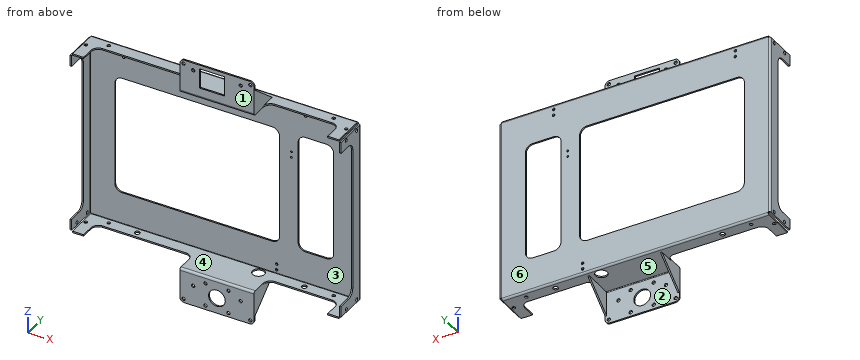
from build123d import *

# Parameters (mm, degrees)
BOSS_EXTRUDE1_DEPTH = 182.5
CUT_EXTRUDE1_DEPTH  = 251
BOSS_EXTRUDE2_START = 17.5
BOSS_EXTRUDE2_DEPTH = 50
BOSS_EXTRUDE3_DEPTH = 2
SKETCH5_R           = 11.25
SKETCH5_R_2         = 2.25
SKETCH5_W           = 34
SKETCH5_H           = 27
CUT_EXTRUDE2_DEPTH  = 2
FILLET1_R           = 10
SKETCH7_W           = 2
SKETCH7_H           = 246
BOSS_EXTRUDE4_DEPTH = 43
SKETCH8_W           = 3
SKETCH8_H           = 3
CUT_EXTRUDE4_DEPTH  = 46
FILLET2_R           = 0.5
FILLET3_R           = 2.5
CUT_EXTRUDE5_DEPTH  = 366
SKETCH10_R          = 2.25
CUT_EXTRUDE6_DEPTH  = 295.5
SKETCH11_R          = 2.25
CUT_EXTRUDE7_DEPTH  = 366
CUT_EXTRUDE8_DEPTH  = 3
SKETCH14_R          = 3.5
SKETCH14_R_2        = 8
CUT_EXTRUDE9_DEPTH  = 10
FILLET4_R           = 6
SKETCH15_R          = 1.75
SKETCH15_R_2        = 1.25
CUT_EXTRUDE10_DEPTH = 10


with BuildPart() as part:
    # Sketch1 → Boss-Extrude1 (new body, symmetric)
    with BuildSketch(Plane(origin=(0, 0, 0), x_dir=(0, 0, -1), z_dir=(1, 0, 0))):
        with BuildLine():
            Line((123, -45), (125, -45))
            Line((125, -45), (125, -2.5))
            ThreePointArc((125, -2.5), (124.267766953, -0.732233047), (122.5, 0))
            Line((122.5, 0), (-122.5, 0))
            ThreePointArc((-122.5, 0), (-124.267766953, -0.732233047), (-125, -2.5))
            Line((-125, -2.5), (-125, -45))
            Line((-125, -45), (-123, -45))
            Line((-123, -45), (-123, -2.5))
            ThreePointArc((-123, -2.5), (-122.853553391, -2.146446609), (-122.5, -2))
            Line((-122.5, -2), (122.5, -2))
            ThreePointArc((122.5, -2), (122.853553391, -2.146446609), (123, -2.5))
            Line((123, -2.5), (123, -45))
        make_face()
    extrude(amount=BOSS_EXTRUDE1_DEPTH, both=True)

    # Sketch2 → Cut-Extrude1 (cut, through all)
    with BuildSketch(Plane(origin=(0, 0, -125), x_dir=(-1, 0, 0), z_dir=(0, 0, -1))):
        with BuildLine():
            Line((-164.5, -45), (164.5, -45))
            Line((164.5, -45), (164.5, -28))
            ThreePointArc((164.5, -28), (161.571067812, -20.928932188), (154.5, -18))
            Line((154.5, -18), (-154.5, -18))
            ThreePointArc((-154.5, -18), (-161.571067812, -20.928932188), (-164.5, -28))
            Line((-164.5, -28), (-164.5, -45))
        make_face()
    extrude(amount=-CUT_EXTRUDE1_DEPTH, mode=Mode.SUBTRACT)

    # Sketch3 → Boss-Extrude2 (add, symmetric)
    with BuildSketch(Plane(origin=(0, 0, 0), x_dir=(0, 0, -1), z_dir=(1, 0, 0)).offset(BOSS_EXTRUDE2_START)):
        with BuildLine():
            Line((-169.5, -47), (-126, -47))
            ThreePointArc((-126, -47), (-125.292893219, -46.707106781), (-125, -46))
            Line((-125, -46), (-125, -18))
            Line((-125, -18), (-123, -18))
            Line((-123, -18), (-123, -46))
            ThreePointArc((-123, -46), (-123.878679656, -48.121320344), (-126, -49))
            Line((-126, -49), (-169.5, -49))
            Line((-169.5, -49), (-169.5, -47))
        make_face()
        with BuildLine():
            Line((126, -47), (169.5, -47))
            Line((169.5, -47), (169.5, -49))
            Line((169.5, -49), (126, -49))
            ThreePointArc((126, -49), (123.878679656, -48.121320344), (123, -46))
            Line((123, -46), (123, -18))
            Line((123, -18), (125, -18))
            Line((125, -18), (125, -46))
            ThreePointArc((125, -46), (125.292893219, -46.707106781), (126, -47))
        make_face()
    extrude(amount=BOSS_EXTRUDE2_DEPTH, both=True)

    # Sketch4 → Boss-Extrude3 (add)
    with BuildSketch(Plane.ZY.offset(32.5)):
        Polygon((125, -7), (158, -47), (125, -47), align=None)
        Polygon((-125, -7), (-158, -47), (-125, -47), align=None)
    boss_extrude3 = extrude(amount=-BOSS_EXTRUDE3_DEPTH)

    # Mirror1: Boss-Extrude3 across plane
    add(boss_extrude3.mirror(Plane(origin=(17.5, 0, 0), x_dir=(0, 0, 1), z_dir=(1, 0, 0))))

    # Sketch5 → Cut-Extrude2 (cut)
    with BuildSketch(Plane.XZ.offset(49)):
        with Locations(Location((17.5, -148.5, 0), (0, 0, 270))):  # turned: the seam where the file's is
            Circle(SKETCH5_R)
        with Locations(Location((2, -133, 0), (0, 0, 270))):  # turned: the seam where the file's is
            Circle(SKETCH5_R_2)
        with Locations(Location((2, -164, 0), (0, 0, 270))):  # turned: the seam where the file's is
            Circle(SKETCH5_R_2)
        with Locations(Location((33, -164, 0), (0, 0, 270))):  # turned: the seam where the file's is
            Circle(SKETCH5_R_2)
        with Locations(Location((33, -133, 0), (0, 0, 270))):  # turned: the seam where the file's is
            Circle(SKETCH5_R_2)
        with Locations(Location((-27.5, -164.5, 0), (0, 0, 270))):  # turned: the seam where the file's is
            Circle(SKETCH5_R_2)
        with Locations(Location((-14.5, -141.85, 0), (0, 0, 270))):  # turned: the seam where the file's is
            Circle(SKETCH5_R_2)
        with Locations(Location((49.5, -141.85, 0), (0, 0, 270))):  # turned: the seam where the file's is
            Circle(SKETCH5_R_2)
        with Locations(Location((-27.5, 164.5, 0), (0, 0, 270))):  # turned: the seam where the file's is
            Circle(SKETCH5_R_2)
        with Locations(Location((-14.5, 159.5, 0), (0, 0, 270))):  # turned: the seam where the file's is
            Circle(SKETCH5_R_2)
        with Locations(Location((49.5, 159.5, 0), (0, 0, 270))):  # turned: the seam where the file's is
            Circle(SKETCH5_R_2)
        with Locations(Location((62.5, -164.5, 0), (0, 0, 270))):  # turned: the seam where the file's is
            Circle(SKETCH5_R_2)
        with Locations(Location((62.5, 164.5, 0), (0, 0, 270))):  # turned: the seam where the file's is
            Circle(SKETCH5_R_2)
        with Locations((11, 151)):
            Rectangle(SKETCH5_W, SKETCH5_H)
    extrude(amount=-CUT_EXTRUDE2_DEPTH, mode=Mode.SUBTRACT)

    # Fillet1
    fillet1_edges = [part.edges().sort_by_distance(p)[0] for p in [
        (-32.5, -18, 124),
        (67.5, -18, 124),
        (-32.5, -18, -124),
        (67.5, -18, -124),
    ]]
    fillet(fillet1_edges, radius=FILLET1_R)

    # Sketch7 → Boss-Extrude4 (add)
    with BuildSketch(Plane.XZ.offset(2)):
        with Locations((-181.5, 0)):
            Rectangle(SKETCH7_W, SKETCH7_H)
        with Locations((181.5, 0)):
            Rectangle(SKETCH7_W, SKETCH7_H)
    extrude(amount=BOSS_EXTRUDE4_DEPTH)

    # Sketch8 → Cut-Extrude4 (cut, through all)
    with BuildSketch(Plane.XZ.offset(45)):
        with Locations((-181, 123.5)):
            Rectangle(SKETCH8_W, SKETCH8_H)
        with Locations((-181, -123.5)):
            Rectangle(SKETCH8_W, SKETCH8_H)
        with Locations((181, -123.5)):
            Rectangle(SKETCH8_W, SKETCH8_H)
        with Locations((181, 123.5)):
            Rectangle(SKETCH8_W, SKETCH8_H)
    extrude(amount=-CUT_EXTRUDE4_DEPTH, mode=Mode.SUBTRACT)

    # Fillet2
    fillet2_edges = [part.edges().sort_by_distance(p)[0] for p in [
        (-180.5, -2, 0),
        (180.5, -2, 0),
    ]]
    fillet(fillet2_edges, radius=FILLET2_R)

    # Fillet3
    fillet3_edges = [part.edges().sort_by_distance(p)[0] for p in [
        (-182.5, 0, 0),
        (182.5, 0, 0),
    ]]
    fillet(fillet3_edges, radius=FILLET3_R)

    # Sketch9 → Cut-Extrude5 (cut, through all)
    with BuildSketch(Plane.ZY.offset(182.5)):
        with BuildLine():
            Line((-107, -45), (107, -45))
            Line((107, -45), (107, -28))
            ThreePointArc((107, -28), (104.071067812, -20.928932188), (97, -18))
            Line((97, -18), (-97, -18))
            ThreePointArc((-97, -18), (-104.071067812, -20.928932188), (-107, -28))
            Line((-107, -28), (-107, -45))
        make_face()
    extrude(amount=-CUT_EXTRUDE5_DEPTH, mode=Mode.SUBTRACT)

    # Sketch10 → Cut-Extrude6 (cut, through all)
    with BuildSketch(Plane.XY.offset(125)):
        with Locations((-175.5, -21)):
            Circle(SKETCH10_R)
        with Locations((-151.5, -9)):
            Circle(SKETCH10_R)
        with Locations((151.5, -9)):
            Circle(SKETCH10_R)
        with Locations((175.5, -21)):
            Circle(SKETCH10_R)
    extrude(amount=-CUT_EXTRUDE6_DEPTH, mode=Mode.SUBTRACT)

    # Sketch11 → Cut-Extrude7 (cut, through all)
    with BuildSketch(Plane.ZY.offset(182.5)):
        with Locations((-118, -9)):
            Circle(SKETCH11_R)
        with Locations((-118, -33)):
            Circle(SKETCH11_R)
        with Locations((118, -9)):
            Circle(SKETCH11_R)
        with Locations((118, -33)):
            Circle(SKETCH11_R)
    extrude(amount=-CUT_EXTRUDE7_DEPTH, mode=Mode.SUBTRACT)

    # Sketch12 → Cut-Extrude8 (cut, through all)
    with BuildSketch(Plane.XZ.offset(2)):
        with BuildLine():
            Line((109.5, 80), (137.5, 80))
            ThreePointArc((137.5, 80), (144.571067812, 77.071067812), (147.5, 70))
            Line((147.5, 70), (147.5, -70))
            ThreePointArc((147.5, -70), (144.571067812, -77.071067812), (137.5, -80))
            Line((137.5, -80), (109.5, -80))
            ThreePointArc((109.5, -80), (102.428932188, -77.071067812), (99.5, -70))
            Line((99.5, -70), (99.5, 70))
            ThreePointArc((99.5, 70), (102.428932188, 77.071067812), (109.5, 80))
        make_face()
        with BuildLine():
            Line((-137.5, 80), (64.5, 80))
            ThreePointArc((64.5, 80), (71.571067812, 77.071067812), (74.5, 70))
            Line((74.5, 70), (74.5, -70))
            ThreePointArc((74.5, -70), (71.571067812, -77.071067812), (64.5, -80))
            Line((64.5, -80), (-137.5, -80))
            ThreePointArc((-137.5, -80), (-144.571067812, -77.071067812), (-147.5, -70))
            Line((-147.5, -70), (-147.5, 70))
            ThreePointArc((-147.5, 70), (-144.571067812, 77.071067812), (-137.5, 80))
        make_face()
    extrude(amount=-CUT_EXTRUDE8_DEPTH, mode=Mode.SUBTRACT)

    # Sketch14 → Cut-Extrude9 (cut)
    with BuildSketch(Plane(origin=(0, 0, -125), x_dir=(-1, 0, 0), z_dir=(0, 0, -1))):
        with Locations((-112.5, -10)):
            Circle(SKETCH14_R)
        with Locations((112.5, -10)):
            Circle(SKETCH14_R)
        with Locations((-51.5, -11)):
            Circle(SKETCH14_R_2)
    extrude(amount=-CUT_EXTRUDE9_DEPTH, mode=Mode.SUBTRACT)

    # Fillet4
    fillet4_edges = [part.edges().sort_by_distance(p)[0] for p in [
        (-32.5, -48, 169.5),
        (67.5, -48, 169.5),
        (-32.5, -48, -169.5),
        (67.5, -48, -169.5),
    ]]
    fillet(fillet4_edges, radius=FILLET4_R)

    # Sketch15 → Cut-Extrude10 (cut)
    with BuildSketch(Plane(origin=(0, 0, 0), x_dir=(1, 0, 0), z_dir=(0, 1, 0))):
        with Locations(Location((109.5, -118, 0), (0, 0, 270))):  # turned: the seam where the file's is
            Circle(SKETCH15_R)
        with Locations(Location((109.5, -110, 0), (0, 0, 270))):  # turned: the seam where the file's is
            Circle(SKETCH15_R)
        with Locations(Location((-135.5, -118, 0), (0, 0, 270))):  # turned: the seam where the file's is
            Circle(SKETCH15_R)
        with Locations(Location((-135.5, -110, 0), (0, 0, 270))):  # turned: the seam where the file's is
            Circle(SKETCH15_R)
        with Locations(Location((70.5, 110, 0), (0, 0, 270))):  # turned: the seam where the file's is
            Circle(SKETCH15_R)
        with Locations(Location((70.5, 118, 0), (0, 0, 270))):  # turned: the seam where the file's is
            Circle(SKETCH15_R)
        with Locations(Location((90.5, -53.8, 0), (0, 0, 270))):  # turned: the seam where the file's is
            Circle(SKETCH15_R_2)
        with Locations(Location((90.5, -45.8, 0), (0, 0, 270))):  # turned: the seam where the file's is
            Circle(SKETCH15_R_2)
    extrude(amount=-CUT_EXTRUDE10_DEPTH, mode=Mode.SUBTRACT)


solid = part.part
The model under review builds one solid part; all positions refer to its coordinate system, in mm. Face numbers are marked on the shaded views. A direction names the side the tool comes from. Give positions to 0.01 mm unless a question says otherwise; leave off trailing zeros. Order: outer loops, then holes, each group sorted by start corner. A loop starts at its lowest first (then second) coordinate and runs counter-clockwise, first axis right, second up. Notation, with made-up numbers: M -14,38 L 45,38 A15 cw 45,59 Z; hole C 52,48.25 d8. An arc over 180 degrees is marked long. One line per question, with ' | ' between items. Start each with the question number.
1) Consider section B-B, the plane z = -148.5. Give the boundary of the cut face in (x, y).
2) Clearance check with flat-ended pins moving along their axes: P1, Ø0.6, axis at x = 175, z = 123.5, coming from the -Y side; P2, Ø1.6, axis at x = 111, z = 123.5, coming from the -Y side; P3, Ø0.9, axis at x = -181.5, y = -33.5, coming from the +Z side. State where each tip first meets the part, or that it passes through.
3) Wall thickness on L1, parallel to Z at x = 4, y = -10.5; L2, parallel to Y at x = 181, z = 118; L3, parallel to X at y = -16.5, z = -88: over which ranges is each line inside the solid? List them lowest first. Write a range as from..to.
4) For the marked faces 3, 4, 5 and 6, list the 3-axis set-ups (+Z, -Z, +X, -X, +Y, -Y) from which the entire face can be reached by the end or side of a thin tool; tool diameter is ignored.
5) Mouldability with a two-part tool opening along X and no side actions: class the marked faces 1 and 2 as pulls with the +X half, pulls with the -X half, needs draft (parallel to the pull), parting line crosses it, or undercut.
6) Consider section C-C, the plane x = 22. State how many separate pieces and enclosed holes the cut face has, then the cut area to 3 significant figures.
7) Consider section A-A, the plane z = -6.5. Give the boundary of the cut face in (x, y).
Found:
1) outline: M -32.5,-49 L 6.25,-49 L 6.25,-47 L -30.5,-47 L -30.5,-35.48 L -32.5,-35.48 Z; M 28.75,-49 L 67.5,-49 L 67.5,-35.48 L 65.5,-35.48 L 65.5,-47 L 28.75,-47 Z
2) P1: stops at y = -45 | P2: stops at y = -18 | P3: stops at z = 122
3) L1: z = -125..-123, 123..125 | L2: y = -45..-35.25, -30.75..-11.25, -6.75..-0.21 | L3: x = -182.5..-180.5, 180.5..182.5
4) face 3: -Y | face 4: +X, -X, -Y | face 5: -Z, +Y | face 6: +Z, -Z, +X, -X, +Y
5) face 1: needs draft | face 2: undercut
6) separate pieces: 4 | enclosed holes: 0 | area: 445 mm²
7) outline: M -182.5,-18 L -180.5,-18 L -180.5,-2.5 A0.5 cw -180,-2 L -147.5,-2 L -147.5,0 L -180,0 A2.5 ccw -182.5,-2.5 Z; M 74.5,-2 L 99.5,-2 L 99.5,0 L 74.5,0 Z; M 147.5,-2 L 180,-2 A0.5 cw 180.5,-2.5 L 180.5,-18 L 182.5,-18 L 182.5,-2.5 A2.5 ccw 180,0 L 147.5,0 Z
